```python
from build123d import *

# Parameters (mm, degrees)
F0_W     = 51.485936
F0_H     = 53.910483
F1_DEPTH = 76.2
F2_SIZE  = 25.4


with BuildPart() as f1:
    # F0 (on Front) → F1 (new body)
    with BuildSketch(Plane.XZ):
        with Locations((-0.249586, 0.463515)):
            Rectangle(F0_W, F0_H)
    extrude(amount=F1_DEPTH)

    # F2
    f2_edges = [f1.edges().sort_by_distance(p)[0] for p in [
        (25.493382, -38.1, 27.418757),
        (-25.992554, -38.1, 27.418757),
        (-0.249586, 0, 27.418757),
        (-0.249586, -76.2, 27.418757),
        (-25.992554, -76.2, 0.463516),
        (-0.249586, -76.2, -26.491726),
        (25.493382, -76.2, 0.463516),
        (-25.992554, -38.1, -26.491726),
        (25.493382, -38.1, -26.491726),
        (-0.249586, 0, -26.491726),
        (25.493382, 0, 0.463516),
    ]]
    chamfer(f2_edges, length=F2_SIZE)


solid = f1.part
```
Source: CAD feature listing. Evaluate the final solid. Frame: model axes, mm. Coordinates: 2 decimals unless noted, no trailing zeros. Order: outer loops, then holes, each group sorted by start corner. A loop starts at its lowest first (then second) coordinate and runs counter-clockwise, first axis right, second up. Notation, with made-up numbers: (-37.5, 15) - (1.5, 15) arc R14 cw to (1.5, 41) - close; hole circle Ø11 at (64.25, 88). An arc over 180 degrees is marked (long way). One line per item, written item: value.
1) Cut plane A-A on y = -28.5. Output: boundary loops of the cut face in (x, z).
Computed values:
outline: (-25.99, -1.09) - (-0.59, -26.49) - (0.09, -26.49) - (25.49, -1.09) - (25.49, 2.02) - (0.09, 27.42) - (-0.59, 27.42) - (-25.99, 2.02) - close
2) Cut plane D-D on z = 9. Output: boundary loops of the cut face in (x, y).
Computed values:
outline: (-19.01, -50.8) - (-0.59, -69.22) - (0.09, -69.22) - (18.51, -50.8) - (18.51, -25.4) - (0.09, -6.98) - (-19.01, -6.98) - close
3) Cut plane C-C on x = -17. Output: boundary loops of the cut face in (y, z).
Computed values:
outline: (-59.79, -1.09) - (-50.8, -10.08) - (-8.99, -10.08) - (0, -1.09) - (0, 2.02) - (-8.99, 11.01) - (-50.8, 11.01) - (-59.79, 2.02) - close
4) Cut plane B-B on z = 19.5. Output: boundary loops of the cut face in (x, y), plus the area to 3 significant figures.
Computed values:
outline: (-8.51, -50.8) - (-0.59, -58.72) - (0.09, -58.72) - (8.01, -50.8) - (8.01, -25.4) - (0.09, -17.48) - (-8.51, -17.48) - close
area: 587 mm^2
5) Contact query for flat-ended pins moving along their axis: pin 1 (8 mm diameter, centred on y = -32.5, z = -6.5, fed in from -X); pin 2 (6 mm diameter, centred on x = 5, z = -10.5, fed in from -Y); pin 3 (8 mm diameter, centred on y = -61, z = -17.5, fed in from +X). Output: stop coordinate, or through.
Computed values:
pin 1: stops at x = -24.58
pin 2: stops at y = -66.13
pin 3: stops at x = 4.54
6) Ray query, line 1 (Y direction, x = -23.5, z = -3); line 2 (Z direction, x = 15.5, y = -47); line 3 (X direction, y = -30.5, z = 11.5). Return the intervals inside material, ascending. Write a range as [from, to].
Computed values:
line 1: y = [-51.38, -1.91]
line 2: z = [-11.09, 12.01]
line 3: x = [-16.51, 16.01]
